Print and shaded views of the part. All mm, measured from the part's lowest x, y and z. A direction names the side the tool comes from. Round coordinates to 2 decimals unless told otherwise and drop trailing zeros. Write each loop counter-clockwise with the first axis right and the second up, starting at its lowest first coordinate (ties: lowest second). Pieces come first, ordered by that corner, then holes. Notation, with made-up numbers: (29.5, 36) - (79.5, 36) arc R24 ccw to (79.5, 74) - close; hole circle Ø11 at (-22, 53.5). An arc over 180 degrees is marked (long way). One line per item, written item: value.
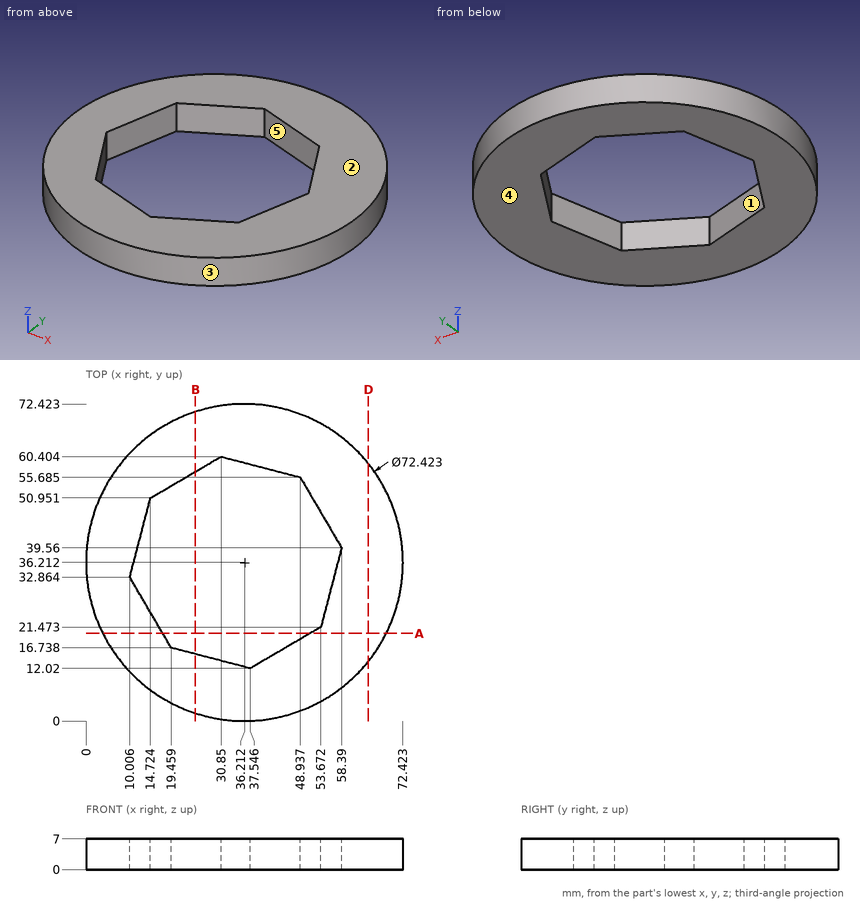
1. Mould opens along Y. For the marked faces 1, 2 and 3 say: released by +Y, released by -Y, zero draft, split by the parting line, or undercut.
Report:
face 1: undercut
face 2: zero draft
face 3: split by the parting line
2. Tool access for the marked faces 4 and 5: list every direction of +Z, -Z, +X, -X, +Y, -Y with a clear straight run to the whole face (end or side of a thin tool).
Report:
face 4: -Z, +X, -X, +Y, -Y
face 5: +Z, -Z
3. Band-saw the part on D-D on x = 64.5. Write the cut outline in (y, z) (1 decimal).
Report:
outline: (13.6, 0) - (58.8, 0) - (58.8, 7) - (13.6, 7) - close
4. Wall check: probe 1 along Y at (x, z) = (46.5, 1); probe 2 along X at (y, z) = (33, 2.5); probe 3 along X at (y, z) = (34.5, 3.75). Give the ranges that are in metal, low to high. Write a range as [from, to].
Report:
probe 1: [1.49, 17.27], [56.32, 70.93]
probe 2: [0.14, 10.04], [56.68, 72.28]
probe 3: [0.04, 10.43], [57.07, 72.38]
5. Band-saw the part on A-A on y = 20. Write the cut outline in (x, z), plus the area to 3 significant figures.
Report:
outline: (3.83, 0) - (17.55, 0) - (17.55, 7) - (3.83, 7) - close; (51.16, 0) - (68.59, 0) - (68.59, 7) - (51.16, 7) - close
area: 218 mm²
6. Drop flat-ended pins along their axis: pin 1 (1.5 mm diameter, centred on x = 19, z = 4, fed in from +Y) (1 decimal); pin 2 (5 mm diameter, centred on x = 52, y = 20, fed in from -Z); pin 3 (1 mm diameter, centred on y = 27.5, z = 1, fed in from +X). Give the stop position or say it passes through.
Report:
pin 1: y = 68.5
pin 2: z = 0
pin 3: x = 71.48
7. Band-saw the part on B-B on x = 25. Write the cut outline in (y, z) (1 decimal), plus the area to 3 significant figures.
Report:
outline: (1.8, 0) - (15.3, 0) - (15.3, 7) - (1.8, 7) - close; (57, 0) - (70.6, 0) - (70.6, 7) - (57, 7) - close
area: 190 mm²
